Autodesk Inventor part; units mm, degrees
ref_plane "YZ Plane" through (0, 0, 0) normal (1, 0, 0) x (0, 1, 0)
ref_plane "XZ Plane" through (0, 0, 0) normal (0, 1, 0) x (-1, 0, 0)
ref_plane "XY Plane" through (0, 0, 0) normal (0, 0, 1) x (1, 0, 0)
sketch "Эскиз4" plane through (0, 0, 0) normal (0, 0, 1) x (1, 0, 0)
  line L0 (-310, 0) -> (-210, 0)
  arc A0 (-210, 0) -> (-155, 25) centre (-210, 73) ccw
  arc A1 (-100, 50) -> (-155, 25) centre (-100, -23) ccw
  line L1 (-100, 50) -> (0, 50)
  line L2 (0, -42.2) -> (0, 92.2)
  line L3 (310, 0) -> (210, 0)
  arc A2 (155, 25) -> (210, 0) centre (210, 73) ccw
  arc A3 (155, 25) -> (100, 50) centre (100, -23) ccw
  line L4 (100, 50) -> (0, 50)
  point P0 (0, 0)
  dimension "d39" = 50
  dimension "d61" = 100
  dimension "d63" = 200
  dimension "d64" = 620
contour flange "Фланец по контуру2" sketch "Эскиз4" thickness 2 bend radius 2 width 70 along (0, 0, 1) mid plane no both sides yes wall seen from (260, 0, 0) lies toward (0, -1, 0) curves L3 A2 A3 L4 L1 A1 A0 L0
bend "Сгиб3"
corner "УглСтык3"
equation "\"d26\" = Толщина"
equation "\"d27\" = Ширина_просечки"
equation "\"d28\" = Глубина_просечки"
equation "\"d29\" = Мин_остаток"
equation "\"d30\" = Радиус_перехода"
equation "\"d32\" = Радиус_гибки"
equation "\"d34\" = Размер_просечки"
equation "\"d35\" = Размер_зазора"
equation "\"d36\" = Радиус_Якоби"
equation "\"Радиус_гибки\" = Толщина"
equation "\"Ширина_просечки\" = Толщина"
equation "\"Глубина_просечки\" = 0.5 * Толщина"
equation "\"Размер_просечки\" = 4 * Толщина"
equation "\"Мин_остаток\" = 2 * Толщина"
equation "\"Радиус_перехода\" = Радиус_гибки"
equation "\"Радиус_Якоби\" = Радиус_гибки"
equation "\"Размер_зазора\" = Толщина"
properties part number "Кожух" material "Алюминий 6061"
For this review, take the finished solid that the model builds, in its own axes (mm). A direction names the side the tool comes from. Coordinates: 2 decimals unless noted, no trailing zeros. Order: outer loops, then holes, each group sorted by start corner. A loop starts at its lowest first (then second) coordinate and runs counter-clockwise, first axis right, second up. Notation, with made-up numbers: (1.5, -9) -> (43.5, -9) arc R17 cw to (43.5, -2) -> close; hole circle Ø11 at (8.25, 62). An arc over 180 degrees is marked (long way). Use CSV: the item, a comma, the result in double quotes. Start each with the question number.
Item 1: We need section A-A, the plane y = 35.5. Give the boundary of the cut face in (x, z), then the cut area to 3 significant figures.
Item 2: For faces 1 (the face through (261, 1, 35)), 2 (the face through (-130.18, 42.37, 34.51)), 3 (the face through (-179.82, 7.63, 34.51)), list the 3-axis set-ups (+Z, -Z, +X, -X, +Y, -Y) from which the entire face can be reached by the end or side of a thin tool; tool diameter is ignored.
Item 3: We need section B-B, the plane z = 43.5. Give the boundary of the cut face in (x, y).
Item 4: Insertion check: pin 1 (21 mm diameter, centred on x = -264, z = 36, fed in from +Y); pin 2 (12 mm diameter, centred on y = 13.5, z = 56, fed in from -X); pin 3 (2 mm diameter, centred on x = -108.5, z = 55.5, fed in from +Y). Each pin has a flat end and moves straight along its axis. Give the tip position at first contact, or say it passes through.
Item 5: Wall thickness on probe 1 along Y at (x, z) = (-271, 49.5); probe 2 along X at (y, z) = (8.5, 48.5); probe 3 along X at (y, z) = (12, 17): over which ranges is each line inside the solid? List them lowest first.
Item 6: Draft analysis for pull direction X (two halves, no side actions). For faces 4 (the face through (-131.023, 44.183, 34.51)), 5 (the face through (-1, 49, 35)), 6 (the face through (-178.977, 5.817, 34.51)), 7 (the face through (-259, 1, 35)), state which applies: pulls with the +X half, pulls with the -X half, needs draft (parallel to the pull), parting line crosses it, or undercut.
Item 7: We need section C-C, the plane x = 230. Give the boundary of the cut face in (y, z), then the cut area to 3 significant figures.
Item 8: We need section D-D, the plane y = 7.5. Give the boundary of the cut face in (x, z), then the cut area to 3 significant figures.
Derived:
1,outline,"(-145.32, 0) -> (-141.97, 0) -> (-141.97, 70) -> (-145.32, 70) -> close; (141.97, 0) -> (145.32, 0) -> (145.32, 70) -> (141.97, 70) -> close"
1,area,"468 mm^2"
2,face 1,"+Z, -Z, +X, +Y"
2,face 2,"+Z, -Z, -Y"
2,face 3,"+Z, -Z, -X, +Y"
3,outline,"(-310, -1) -> (-210, -1) arc R74 ccw to (-154.25, 24.34) arc R72 cw to (-100, 49) -> (100, 49) arc R72 cw to (154.25, 24.34) arc R74 ccw to (210, -1) -> (310, -1) -> (310, 1) -> (210, 1) arc R72 cw to (155.75, 25.66) arc R74 ccw to (100, 51) -> (-100, 51) arc R74 ccw to (-155.75, 25.66) arc R72 cw to (-210, 1) -> (-310, 1) -> close"
4,pin 1,"stops at y = 1"
4,pin 2,"stops at x = -180.1"
4,pin 3,"stops at y = 50.62"
5,probe 1,"y = -1 to 1"
5,probe 2,"x = -178 to -173.73, 173.73 to 178"
5,probe 3,"x = -171.75 to -168.11, 168.11 to 171.75"
6,face 4,"pulls with the -X half"
6,face 5,"undercut"
6,face 6,"undercut"
6,face 7,"needs draft"
7,outline,"(-1, 0) -> (1, 0) -> (1, 70) -> (-1, 70) -> close"
7,area,"140 mm^2"
8,outline,"(-180.1, 0) -> (-175.57, 0) -> (-175.57, 70) -> (-180.1, 70) -> close; (175.57, 0) -> (180.1, 0) -> (180.1, 70) -> (175.57, 70) -> close"
8,area,"635 mm^2"
